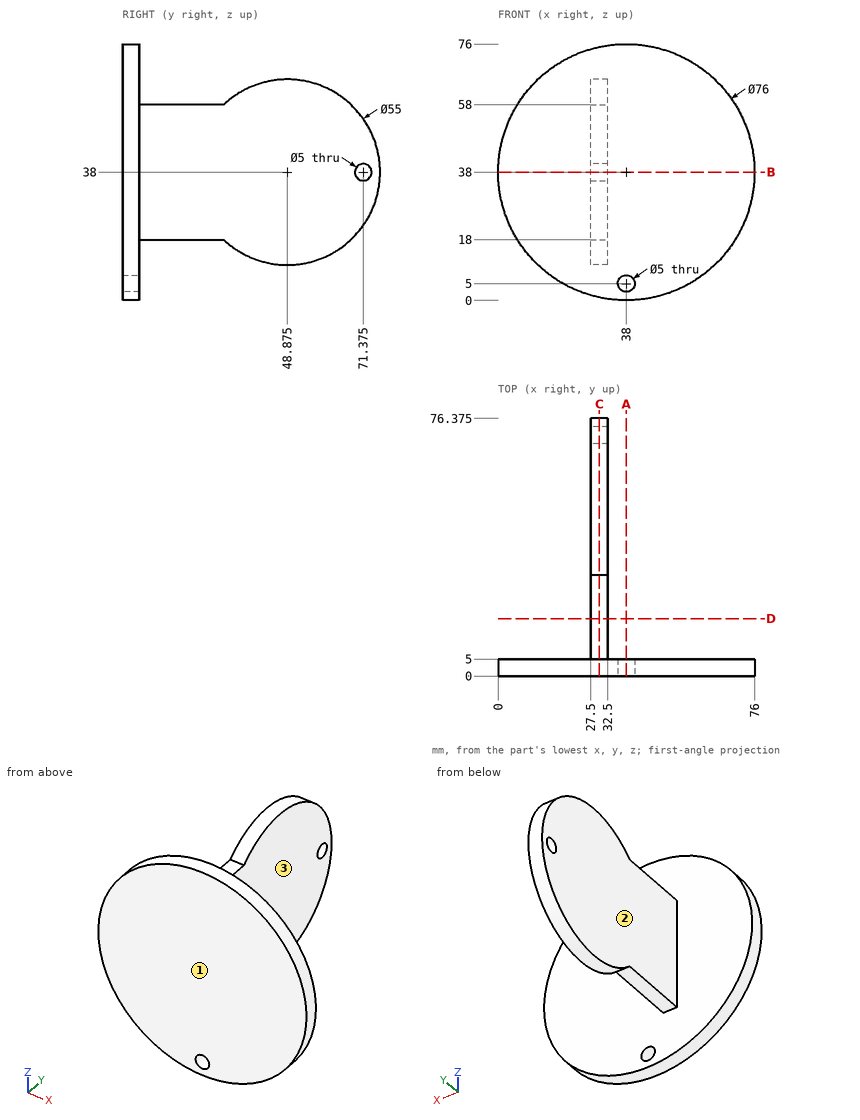
Here's the drawing with two shaded views (mm, measured from the low corner). I have some questions. A direction names the side the tool comes from. Give positions to 0.01 mm unless a question says otherwise; leave off trailing zeros. Order: outer loops, then holes, each group sorted by start corner. A loop starts at its lowest first (then second) coordinate and runs counter-clockwise, first axis right, second up.
Q1. Suppose I cut it at C-C, the plane x = 30. Write out the boundary of the cut face in (y, z) (1 decimal).
Q2. If I drill on line 1 along Y through (x, z) = (24, 24); line 2 along X through (y, z) = (54, 23); line 3 along X through (y, z) = (1.45, 5) (1 decimal), over which ranges is the centre line in solid material (lowest first)?
Q3. For the marked faces 1, 2 and 3, which set-ups out of +Z, -Z, +X, -X, +Y, -Y let a thin tool reach every point of the face, with its end or its side?
Q4. I'm going to push flat-ended pins straight in: P1, Ø1.5, axis at x = 38.5, z = 56, coming from the +Y side; P2, Ø4, axis at x = 29, y = 14.5, coming from the +Z side; P3, Ø4, axis at y = 22.5, z = 46, coming from the -X side. Where does each tip first touch, or does it pass through?
Q5. Suppose I cut it at D-D, the plane y = 17. Write out the boundary of the cut face in (x, z).
Q6. Suppose I cut it at B-B, the plane z = 38. Write out the boundary of the cut face in (x, y) (1 decimal), and give its area (3 significant figures).
Q7. Suppose I cut it at A-A, the plane x = 38. Write out the boundary of the cut face in (y, z).
Solution:
1. outline: (0, 0.9) - (5, 0.9) - (5, 18) - (30, 18) arc R27.5 ccw (long way) to (30, 58) - (5, 58) - (5, 75.1) - (0, 75.1) - close; hole circle Ø5 at (71.4, 38)
2. line 1: y = 0 to 5
2. line 2: x = 27.5 to 32.5
2. line 3: x = 19.2 to 35.5, 40.5 to 56.8
3. face 1: +Z, -Z, +X, -X, -Y
3. face 2: +Z, -Z, -X, +Y
3. face 3: +Z, -Z, +X, +Y
4. P1: stops at y = 5
4. P2: stops at z = 58
4. P3: stops at x = 27.5
5. outline: (27.5, 18) - (32.5, 18) - (32.5, 58) - (27.5, 58) - close
6. outline: (0, 0) - (76, 0) - (76, 5) - (32.5, 5) - (32.5, 68.9) - (27.5, 68.9) - (27.5, 5) - (0, 5) - close; (27.5, 73.9) - (32.5, 73.9) - (32.5, 76.4) - (27.5, 76.4) - close
6. area: 712 mm2
7. outline: (0, 0) - (5, 0) - (5, 2.5) - (0, 2.5) - close; (0, 7.5) - (5, 7.5) - (5, 76) - (0, 76) - close
